```python
from build123d import *

# Parameters (mm, degrees)
SKETCH1_R           = 85
BOSS_EXTRUDE1_DEPTH = 19
SKETCH2_R           = 17.5
CUT_EXTRUDE1_DEPTH  = 122.70045193
SKETCH3_R           = 10
CUT_EXTRUDE2_DEPTH  = 14.761809
CIRPATTERN1_START   = 4.238190927
CIRPATTERN1_DEPTH   = 14.761809073


# Read off the part's stored shape, not the designer's step: CirPattern1
with BuildPart() as part:
    # Sketch1 → Boss-Extrude1 (new body)
    with BuildSketch(Plane(origin=(0, 0, 0), x_dir=(1, 0, 0), z_dir=(0, 1, 0))):
        with Locations(Location((0, 0, 0), (0, 0, 270))):
            Circle(SKETCH1_R)
    extrude(amount=BOSS_EXTRUDE1_DEPTH)

    # Sketch2 → Cut-Extrude1 (cut, through all)
    with BuildSketch(Plane(origin=(0, 0, 0), x_dir=(1, 0, 0), z_dir=(0, 1, 0))):
        with Locations(Location((0, 0, 0), (0, 0, 270))):
            Circle(SKETCH2_R)
    extrude(amount=CUT_EXTRUDE1_DEPTH, mode=Mode.SUBTRACT)

    # Sketch3 → Cut-Extrude2 (cut)
    with BuildSketch(Plane(origin=(0, 19, 0), x_dir=(1, 0, 0), z_dir=(0, 1, 0))):
        with Locations((-23.395464248, 0)):
            Circle(SKETCH3_R)
    extrude(amount=-CUT_EXTRUDE2_DEPTH, mode=Mode.SUBTRACT)

    # CirPattern1 outline → CirPattern1 (cut)
    with BuildSketch(Plane(origin=(0, 0, 0), x_dir=(1, 0, 0), z_dir=(0, 1, 0)).offset(CIRPATTERN1_START)):
        with BuildLine():
            ThreePointArc((-16.105637815, -6.845321802), (-19.742724386, -9.309000564), (-24.084720779, -9.976217992))
            ThreePointArc((-24.084720779, -9.976217992), (-23.614159231, -23.614159231), (-9.976217993, -24.084720779))
            ThreePointArc((-9.976217993, -24.084720779), (0, -33.395464248), (9.976217993, -24.084720779))
            ThreePointArc((9.976217993, -24.084720779), (23.614159231, -23.614159231), (24.084720779, -9.976217993))
            ThreePointArc((24.084720779, -9.976217993), (33.395464248, 0), (24.084720779, 9.976217993))
            ThreePointArc((24.084720779, 9.976217993), (23.614159231, 23.614159231), (9.976217993, 24.084720779))
            ThreePointArc((9.976217993, 24.084720779), (0, 33.395464248), (-9.976217993, 24.084720779))
            ThreePointArc((-9.976217993, 24.084720779), (-23.614159231, 23.614159231), (-24.084720779, 9.976217993))
            ThreePointArc((-24.084720779, 9.976217993), (-19.742724386, 9.309000564), (-16.105637815, 6.845321802))
            ThreePointArc((-16.105637815, 6.845321802), (17.5, 0), (-16.105637815, -6.845321802))
        make_face()
    extrude(amount=CIRPATTERN1_DEPTH, mode=Mode.SUBTRACT)


solid = part.part
```
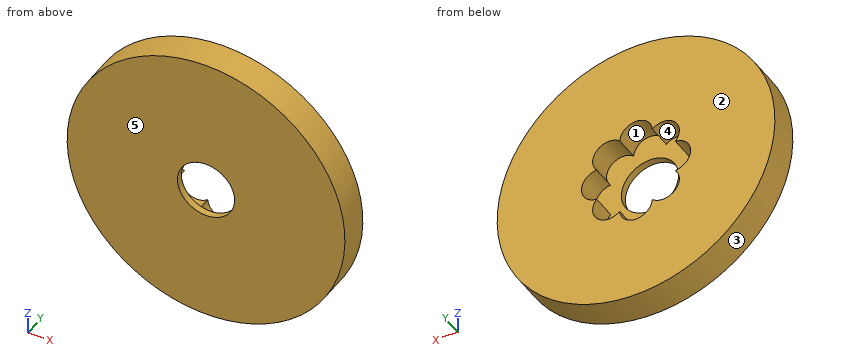
The listing builds one solid part. Answer for the finished solid, in the listing's coordinates (mm). Face numbers are marked on the shaded views. A direction names the side the tool comes from. Give positions to 0.01 mm unless a question says otherwise; leave off trailing zeros. Order: outer loops, then holes, each group sorted by start corner. A loop starts at its lowest first (then second) coordinate and runs counter-clockwise, first axis right, second up. Notation, with made-up numbers: (51, 18) -> (97, 18) arc R13 ccw to (97, 39) -> close; hole circle Ø8 at (-6.5, 72.5). An arc over 180 degrees is marked (long way). Answer as CSV lines item,"result". Start each with the question number.
Q1. A cutting plane is placed at D-D (z = 22). Determine the outline of the cut face in (x, y), then the cut area to 3 significant figures.
Q2. A cutting plane is placed at C-C (y = 15.5). Determine the outline of the cut face in (x, z).
Q3. Determine the mould class of the marked faces 1, 2 and 3 for opening direction Z: pulls with the +Z half, pulls with the -Z half, needs draft (parallel to the pull), parting line crosses it, or undercut.
Q4. A cutting plane is placed at A-A (x = 0). Determine the outline of the cut face in (y, z).
Q5. Given pin 1 (3 mm diameter, centred on y = 16, z = 61.5, fed in from +X); pin 2 (4 mm diameter, centred on y = 8.5, z = 55.5, fed in from +X); pin 3 (1.5 mm diameter, centred on x = -13.5, y = 7, fed in from -Z), each flat-ended and moving along its own axis, determine where each tip first touches the part or whether it passes through.
Q6. Find the intervals of material crossed by L1, parallel to X at y = 2.65, z = 0; L2, parallel to Y at x = -11.5, z = -15.5; L3, parallel to X at y = 9.75, z = -18, in increasing order.
Q7. A cutting plane is placed at B-B (z = 0). Determine the outline of the cut face in (x, y), then the cut area to 3 significant figures.
Q8. Which of the six approach directions +Z, -Z, +X, -X, +Y, -Y give full straight-line access (tool end or side, diameter ignored) to the marked faces 4 and 5?
Results found:
1,outline,"(-82.1, 0) -> (82.1, 0) -> (82.1, 19) -> (24.92, 19) -> (24.92, 4.24) -> (-24.92, 4.24) -> (-24.92, 19) -> (-82.1, 19) -> close"
1,area,"2,380 mm2"
2,outline,"circle Ø170 at (0, 0); hole (-24.08, -9.98) arc R10 ccw to (-9.98, -24.08) arc R10 ccw to (9.98, -24.08) arc R10 ccw to (24.08, -9.98) arc R10 ccw to (24.08, 9.98) arc R10 ccw to (9.98, 24.08) arc R10 ccw to (-9.98, 24.08) arc R10 ccw to (-24.08, 9.98) arc R10 ccw to start"
3,face 1,"undercut"
3,face 2,"needs draft"
3,face 3,"parting line crosses it"
4,outline,"(0, -85) -> (19, -85) -> (19, -33.4) -> (4.24, -33.4) -> (4.24, -17.5) -> (0, -17.5) -> close; (0, 17.5) -> (4.24, 17.5) -> (4.24, 33.4) -> (19, 33.4) -> (19, 85) -> (0, 85) -> close"
5,pin 1,"x = 60.21"
5,pin 2,"x = 66.05"
5,pin 3,"z = -84.04"
6,L1,"-85 to -17.5, 17.5 to 85"
6,L2,"0 to 4.24"
6,L3,"-83.07 to -26.44, 26.44 to 83.07"
7,outline,"(-85, 0) -> (-17.5, 0) -> (-17.5, 4.24) -> (-33.4, 4.24) -> (-33.4, 19) -> (-85, 19) -> close; (17.5, 0) -> (85, 0) -> (85, 19) -> (33.4, 19) -> (33.4, 4.24) -> (17.5, 4.24) -> close"
7,area,"2,100 mm2"
8,face 4,"+Y"
8,face 5,"+Z, -Z, +X, -X, -Y"
